```python
from build123d import *

# Parameters (mm, degrees)
BOSS_EXTRUDE1_DEPTH        = 42
M18X1_5_TAPPED_HOLE1_D     = 16.5
M18X1_5_TAPPED_HOLE1_DEPTH = 43.5
M18X1_5_TAPPED_HOLE1_TIP   = 4.957100107


with BuildPart() as part:
    # Sketch1 → Boss-Extrude1 (new body)
    with BuildSketch(Plane.XY):
        Polygon((-30, 15), (15, 35), (30, 35), (30, -15), (-30, -15), align=None)
    extrude(amount=BOSS_EXTRUDE1_DEPTH)

    # M18x1.5 Tapped Hole1
    with Locations(Plane(origin=(30, 10, 21), x_dir=(0, 1, 0), z_dir=(1, 0, 0))):
        with Locations((0, 0)):
            Hole(M18X1_5_TAPPED_HOLE1_D / 2, depth=M18X1_5_TAPPED_HOLE1_DEPTH)
            with Locations((0, 0, -(M18X1_5_TAPPED_HOLE1_DEPTH + M18X1_5_TAPPED_HOLE1_TIP / 2))):  # 118° drill point
                Cone(0, M18X1_5_TAPPED_HOLE1_D / 2, M18X1_5_TAPPED_HOLE1_TIP, mode=Mode.SUBTRACT)


solid = part.part
```
The model under review builds one solid part; all positions refer to its coordinate system, in mm. A direction names the side the tool comes from. Give positions to 0.01 mm unless a question says otherwise; leave off trailing zeros. Loops run counter-clockwise (first coordinate to the right, second up) from the corner with the lowest first, then second, coordinate; pieces in that order, holes last. Notation, with made-up numbers: (41, 87.5) - (100, 87.5) arc R37 ccw to (100, 123.5) - close; hole circle Ø2 at (-16, 12.25). An arc over 180 degrees is marked (long way). Answer as a JSON object with one key per item and string values.
Q1. Add section D-D on x = -14.5. State the section outline as (y, z) points, plus the area to 3 significant figures.
Worked out:
{"outline": "(-15, 0) - (21.89, 0) - (21.89, 42) - (-15, 42) - close; hole circle Ø13.17 at (10, 21)", "area": "1,410 mm^2"}
Q2. Mouldability with a two-part tool opening along Y and no side actions: class faces 3 (the flat face through (0, 5, 0)), 4 (the conical face through (-17.596, 9.689, 19.601)), 5 (the flat face through (22, 35, 21)) as +Y half, -Y half, draft (parallel to the pull), parting line (faces both ways), or undercut.
Worked out:
{"face 3": "draft", "face 4": "undercut", "face 5": "+Y half"}
Q3. Add section C-C on y = 31. State the section outline as (x, z) points, plus the area to 3 significant figures.
Worked out:
{"outline": "(6, 0) - (30, 0) - (30, 42) - (6, 42) - close", "area": "1,010 mm^2"}
Q4. Insertion check: pin 1 (19 mm diameter, centred on y = 10, z = 21, fed in from +X); pin 2 (1.5 mm diameter, centred on x = 9, z = 13, fed in from +Y); pin 3 (2 mm diameter, centred on y = 6.5, z = 26.5, fed in from +X). Each pin has a flat end and moves straight along its axis. Give the tip position at first contact, or say it passes through.
Worked out:
{"pin 1": "stops at x = 30", "pin 2": "stops at y = 32.67", "pin 3": "stops at x = -13.94"}
Q5. Add section B-B on x = -4. State the section outline as (y, z) points, plus the area to 3 significant figures.
Worked out:
{"outline": "(-15, 0) - (26.56, 0) - (26.56, 42) - (-15, 42) - close; hole circle Ø16.5 at (10, 21)", "area": "1,530 mm^2"}
Q6. To check wall thickness, follow line 1 along Z through (x, y) = (18, 10); line 2 along Y through (x, z) = (6, 21); line 3 along Y through (x, z) = (12, 14.5). State the ranges of each line that lie inside material, in increasing order.
Worked out:
{"line 1": "z = 0 to 12.75, 29.25 to 42", "line 2": "y = -15 to 1.75, 18.25 to 31", "line 3": "y = -15 to 4.92, 15.08 to 33.67"}
Q7. For faces 1 (the cylindrical face through (7.945, 6.193, 13.681)), 2 (the flat face through (-30, 0, 21)), list the 3-axis set-ups (+Z, -Z, +X, -X, +Y, -Y) from which the entire face can be reached by the end or side of a thin tool; tool diameter is ignored.
Worked out:
{"face 1": "+X", "face 2": "+Z, -Z, -X, +Y, -Y"}
Q8. Add section A-A on z = 33.5. State the section outline as (x, y) points, plus the area to 3 significant figures.
Worked out:
{"outline": "(-30, -15) - (30, -15) - (30, 35) - (15, 35) - (-30, 15) - close", "area": "2,550 mm^2"}
